Read the model definition and answer for the solid it produces. Units are mm, in the model's axes. A direction names the side the tool comes from. Give positions to 0.01 mm unless a question says otherwise; leave off trailing zeros. Write each loop counter-clockwise with the first axis right and the second up, starting at its lowest first coordinate (ties: lowest second). Pieces come first, ordered by that corner, then holes. Notation, with made-up numbers: M 55,64.5 L 86,64.5 A26 cw 86,79.5 Z; hole C 78,23 d3. An arc over 180 degrees is marked long. Write each question's results on one line, items separated by ' | '. Start each with the question number.
```python
from build123d import *

# Parameters (mm, degrees)
F0_W     = 63.5
F0_H     = 203.2
F1_DEPTH = 7.62
F3_DEPTH = 12.7
F4_W     = 2.3368
F4_H     = 25.4
F4_W_2   = 2.338178
F5_DEPTH = 25.4


with BuildPart() as f1:
    # F0 (on Top) → F1 (new body)
    with BuildSketch(Plane.XY):
        with Locations((-31.75, 26.023151)):
            Rectangle(F0_W, F0_H)
    extrude(amount=F1_DEPTH)

    # F2 (on face) → F3 (cut)
    with BuildSketch(Plane.XY.offset(7.62)):
        Polygon((-19.05, -59.665699), (-19.05, -12.076849), (-31.75, -12.076849), (-44.45, -12.076849), (-44.45, -59.665699), align=None)
    extrude(amount=-F3_DEPTH, mode=Mode.SUBTRACT)

    # F4 (on face) → F5 (cut)
    with BuildSketch(Plane.XY.offset(7.62)):
        with Locations((-57.605822, 107.303151)):
            Rectangle(F4_W, F4_H)
        with Locations((-57.606511, -45.096849)):
            Rectangle(F4_W_2, F4_H)
        with Locations((-5.894178, 107.303151)):
            Rectangle(F4_W, F4_H)
        with Locations((-5.893489, -45.096849)):
            Rectangle(F4_W_2, F4_H)
    extrude(amount=-F5_DEPTH, mode=Mode.SUBTRACT)


solid = f1.part
```
Item 1: For faces 5 (the flat face through (-32, 127.623, 4)), 6 (the flat face through (-7.063, 107, 4)), determine the directions among +Z, -Z, +X, -X, +Y, -Y from which every point of the face is accessible in a straight line to the end or side of a thin tool.
Item 2: Determine the mould class of faces 1 (the flat face through (-32, 27, 7.62)), 2 (the flat face through (-63.5, 25, 4)), 3 (the flat face through (-32, -59.666, 4)), 4 (the flat face through (0, 25, 4)) for opening direction X: +X half, -X half, draft (parallel to the pull), parting line (faces both ways), or undercut.
Item 3: Section C-C, the plane x = -21 is taken. Determine the outline of the cut face in (y, z).
Item 4: Straight lines are drawn through the part: line 1 (X direction, y = 101.5, z = 4); line 2 (Y direction, x = -58, z = 5.5); line 3 (Y direction, x = -34.5, z = 6.75). For each, find the intervals that lie inside material, in ascending order.
Item 5: Section B-B, the plane z = 1.75 is taken. Determine the outline of the cut face in (x, y), then the cut area to 3 significant figures.
Item 6: Section D-D, the plane y = -14 is taken. Determine the outline of the cut face in (x, z), then the cut area to 3 significant figures.
Item 7: Section A-A, the plane y = 97 is taken. Determine the outline of the cut face in (x, z), then the cut area to 3 significant figures.
Item 8: Given P1, Ø4, axis at x = -23, y = 99.5, coming from the -Z side, flat-ended and moving along its own axis, determine where the tip first touches the part or whether it passes through.
Worked out:
1) face 5: +Z, -Z, +X, -X, +Y | face 6: +Z, -Z
2) face 1: draft | face 2: -X half | face 3: undercut | face 4: +X half
3) outline: M -75.58,0 L -59.67,0 L -59.67,7.62 L -75.58,7.62 Z; M -12.08,0 L 127.62,0 L 127.62,7.62 L -12.08,7.62 Z
4) line 1: x = -63.5 to -58.77, -56.44 to -7.06, -4.73 to 0 | line 2: y = -75.58 to -57.8, -32.4 to 94.6, 120 to 127.62 | line 3: y = -75.58 to -59.67, -12.08 to 127.62
5) outline: M -63.5,-75.58 L 0,-75.58 L 0,127.62 L -63.5,127.62 Z; hole M -58.78,-57.8 L -56.44,-57.8 L -56.44,-32.4 L -58.78,-32.4 Z; hole M -58.77,94.6 L -56.44,94.6 L -56.44,120 L -58.77,120 Z; hole M -44.45,-59.67 L -19.05,-59.67 L -19.05,-12.08 L -44.45,-12.08 Z; hole M -7.06,-57.8 L -4.72,-57.8 L -4.72,-32.4 L -7.06,-32.4 Z; hole M -7.06,94.6 L -4.73,94.6 L -4.73,120 L -7.06,120 Z | area: 11,500 mm²
6) outline: M -63.5,0 L -44.45,0 L -44.45,7.62 L -63.5,7.62 Z; M -19.05,0 L 0,0 L 0,7.62 L -19.05,7.62 Z | area: 290 mm²
7) outline: M -63.5,0 L -58.77,0 L -58.77,7.62 L -63.5,7.62 Z; M -56.44,0 L -7.06,0 L -7.06,7.62 L -56.44,7.62 Z; M -4.73,0 L 0,0 L 0,7.62 L -4.73,7.62 Z | area: 448 mm²
8) P1: stops at z = 0
